from build123d import *

# Parameters (mm, degrees)
SKETCH1_R           = 3.175
BOSS_EXTRUDE1_DEPTH = 10
SKETCH3_R           = 3.275
CUT_EXTRUDE1_DEPTH  = 7.5
CIRPATTERN1_COUNT   = 3


with BuildPart() as part:
    # Sketch1 → Boss-Extrude1 (new body)
    # profile 1 of 4: a face of its own
    with BuildSketch(Plane(origin=(0, 0, 0), x_dir=(1, 0, 0), z_dir=(0, 1, 0))):
        with BuildLine():
            ThreePointArc((-14.698323484, 16.673963027), (-22.2275, 0), (-14.698323484, -16.673963027))
            ThreePointArc((-14.698323484, -16.673963027), (-12.11375, -20.98163047), (-7.090913821, -21.066103043))
            ThreePointArc((-7.090913821, -21.066103043), (11.11375, -19.249579663), (21.789237305, -4.392140016))
            ThreePointArc((21.789237305, -4.392140016), (24.2275, 0), (21.789237305, 4.392140016))
            ThreePointArc((21.789237305, 4.392140016), (11.11375, 19.249579663), (-7.090913821, 21.066103043))
            ThreePointArc((-7.090913821, 21.066103043), (-12.11375, 20.98163047), (-14.698323484, 16.673963027))
        make_face()
        with Locations((-9.52625, 16.499949006)):
            Circle(SKETCH1_R, mode=Mode.SUBTRACT)
        with Locations((19.0525, 0)):
            Circle(SKETCH1_R, mode=Mode.SUBTRACT)
        with Locations((-9.52625, -16.499949006)):
            Circle(SKETCH1_R, mode=Mode.SUBTRACT)
        with BuildLine():
            ThreePointArc((-4.511236152, -15.223132222), (7.93875, -13.750318349), (15.439237305, -3.704721001))
            ThreePointArc((15.439237305, -3.704721001), (13.8775, 0), (15.439237305, 3.704721001))
            ThreePointArc((15.439237305, 3.704721001), (7.93875, 13.750318349), (-4.511236152, 15.223132222))
            ThreePointArc((-4.511236152, 15.223132222), (-6.93875, 12.018267541), (-10.928001153, 11.518411221))
            ThreePointArc((-10.928001153, 11.518411221), (-15.8775, 0), (-10.928001153, -11.518411221))
            ThreePointArc((-10.928001153, -11.518411221), (-6.93875, -12.018267541), (-4.511236152, -15.223132222))
        make_face(mode=Mode.SUBTRACT)
    # profile 2 of 4: a face of its own
    with BuildSketch(Plane(origin=(0, 0, 0), x_dir=(1, 0, 0), z_dir=(0, 1, 0))):
        with Locations((19.0525, 0)):
            Circle(SKETCH1_R)
    # profile 3 of 4: a face of its own
    with BuildSketch(Plane(origin=(0, 0, 0), x_dir=(1, 0, 0), z_dir=(0, 1, 0))):
        with Locations((-9.52625, 16.499949006)):
            Circle(SKETCH1_R)
    # profile 4 of 4: a face of its own
    with BuildSketch(Plane(origin=(0, 0, 0), x_dir=(1, 0, 0), z_dir=(0, 1, 0))):
        with Locations((-9.52625, -16.499949006)):
            Circle(SKETCH1_R)
    extrude(amount=BOSS_EXTRUDE1_DEPTH)

    # Sketch3 → Cut-Extrude1 (cut)
    with BuildSketch(Plane(origin=(0, 10, 0), x_dir=(1, 0, 0), z_dir=(0, 1, 0))):
        with Locations(Location((19.0525, 0, 0), (0, 0, 270))):
            Circle(SKETCH3_R)
    cut_extrude1 = extrude(amount=-CUT_EXTRUDE1_DEPTH, mode=Mode.SUBTRACT)

    # CirPattern1: Cut-Extrude1 ×3 about axis
    cirpattern1_axis = Axis((0, 0, 0), (0, 1, 0))
    for i in range(1, CIRPATTERN1_COUNT):
        add(cut_extrude1.rotate(cirpattern1_axis, i * 360 / CIRPATTERN1_COUNT), mode=Mode.SUBTRACT)


solid = part.part
The model under review builds one solid part; all positions refer to its coordinate system, in mm. A direction names the side the tool comes from. Round coordinates to 2 decimals unless told otherwise and drop trailing zeros. Order: outer loops, then holes, each group sorted by start corner. A loop starts at its lowest first (then second) coordinate and runs counter-clockwise, first axis right, second up. Notation, with made-up numbers: (68.5, 1.5) -> (80.5, 1.5) arc R19 cw to (80.5, 28.5) -> close; hole circle Ø6 at (86.25, 88.25). An arc over 180 degrees is marked (long way). Write item = value, one per line. Start each with the question number.
Item 1: Consider section D-D on y = 6.75. Count the separate pieces of the cut face and the enclosed holes in it, plus the area to 3 significant figures.
Item 2: Mouldability with a two-part tool opening along Z and no side actions: class faces 4 (the face through (-12.05, 4.93, -21.02)), 5 (the face through (16, 0, 0)), 6 (the face through (-6.99, 4.93, 11.99)) as released by +Z, released by -Z, zero draft, split by the parting line, or undercut.
Item 3: Consider section B-B on x = 7. Write out the cut boundary in (y, z), plus the area to 3 significant figures.
Item 4: Consider section A-A on z = 0. Write out the cut boundary in (x, y).
Item 5: For line 1 along X through (y, z) = (7, 0); line 2 along X through (y, z) = (9.5, 2); line 3 along Z through (x, y) = (-0.5, 8.75), list the stretches that pass through material, from the lowest coordinate up.
Item 6: For faces 1 (the face through (10.884, 4.93, 19.38)), 2 (the face through (-8.543, 6.302, -13.376)), 3 (the face through (7.78, 4.93, 13.84)), list the 3-axis set-ups (+Z, -Z, +X, -X, +Y, -Y) from which the entire face can be reached by the end or side of a thin tool; tool diameter is ignored.
Item 7: Clearance check with flat-ended pins moving along their axes: pin 1 Ø6 at (x, z) = (-9.53, -16.5) entering from +Y; pin 2 Ø6 at (y, z) = (1, -4.5) entering from -X; pin 3 Ø5 at (x, y) = (-5.5, 5) entering from -Z. State where each tip first meets the part, or that it passes through.
Conclusion:
q1.separate_pieces = 1
q1.enclosed_holes = 4
q1.area = 727 mm2
q2.face_4 = released by -Z
q2.face_5 = zero draft
q2.face_6 = undercut
q3.outline = (0, -21.1) -> (10, -21.1) -> (10, -14.25) -> (0, -14.25) -> close; (0, 14.25) -> (10, 14.25) -> (10, 21.1) -> (0, 21.1) -> close
q3.area = 137 mm2
q4.outline = (-22.23, 0) -> (-15.88, 0) -> (-15.88, 10) -> (-22.23, 10) -> close; (13.88, 0) -> (24.23, 0) -> (24.23, 10) -> (22.33, 10) -> (22.33, 2.5) -> (15.78, 2.5) -> (15.78, 10) -> (13.88, 10) -> close
q5.line_1 = -22.23 to -15.88, 13.88 to 15.78, 22.33 to 24.23
q5.line_2 = -22.14 to -15.75, 14.28 to 16.46, 21.65 to 23.83
q5.line_3 = -22.22 to -15.87, 15.87 to 22.22
q6.face_1 = +Z, +Y, -Y
q6.face_2 = +Y
q6.face_3 = +Y, -Y
q7.pin_1 = 2.5
q7.pin_2 = -22.18
q7.pin_3 = -22.02
